For this review, take the finished solid that the model builds, in its own axes (mm). Round coordinates to 2 decimals unless told otherwise and drop trailing zeros. Order: outer loops, then holes, each group sorted by start corner. A loop starts at its lowest first (then second) coordinate and runs counter-clockwise, first axis right, second up. Notation, with made-up numbers: (-13.75, 1) -> (24.25, 1) arc R27 ccw to (24.25, 38) -> close; hole circle Ø11 at (4, -20.75). An arc over 180 degrees is marked (long way). Put each result on its own line as item: value. Start each with the question number.
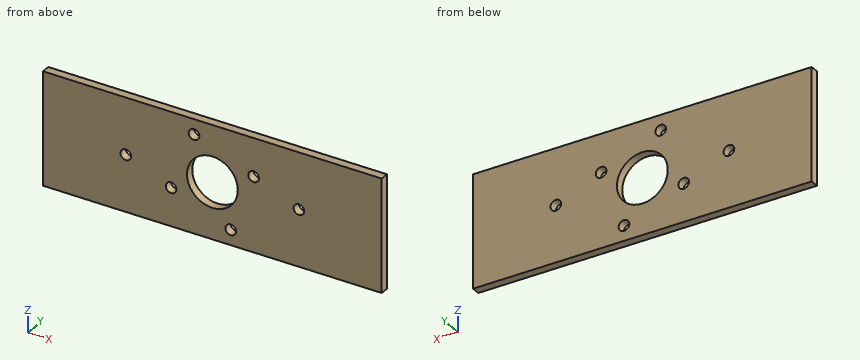
```python
from build123d import *

# Parameters (mm, degrees)
SKETCH1_W                = 190.5
SKETCH1_H                = 63.5
BOSS_EXTRUDE1_DEPTH      = 4.7625
SKETCH3_R                = 14.2875
CUT_EXTRUDE1_DEPTH       = 101.515204851
F_6_0_6_DIAMETER_HOLE1_D = 6


with BuildPart() as part:
    # Sketch1 → Boss-Extrude1 (new body)
    with BuildSketch(Plane(origin=(0, 0, 0), x_dir=(1, 0, 0), z_dir=(0, 1, 0))):
        Rectangle(SKETCH1_W, SKETCH1_H)
    extrude(amount=BOSS_EXTRUDE1_DEPTH)

    # Sketch3 → Cut-Extrude1 (cut, through all)
    with BuildSketch(Plane(origin=(0, 4.7625, 0), x_dir=(1, 0, 0), z_dir=(0, 1, 0))):
        with Locations(Location((0, 0, 0), (0, 0, 270))):
            Circle(SKETCH3_R)
    extrude(amount=-CUT_EXTRUDE1_DEPTH, mode=Mode.SUBTRACT)

    # Ø6.0 (6) Diameter Hole1 (through all)
    with Locations(Plane(origin=(0, 4.7625, 0), x_dir=(1, 0, 0), z_dir=(0, 1, 0))):
        with Locations((-23.209797391, 10.318202609), (-10.318202609, -23.209797391), (10.318202609, 23.209797391), (23.209797391, -10.318202609), (-48.683333333, 0), (48.683333333, 0)):
            Hole(F_6_0_6_DIAMETER_HOLE1_D / 2)


solid = part.part
```
Item 1: Consider section A-A, the plane z = 0. Write out the cut boundary in (x, y).
Item 2: For L1, parallel to Z at x = 1, y = 1.55; L2, parallel to X at y = 3.6, z = 2.5; L3, parallel to X at y = 4.35, z = -10, list the stretches that pass through material, from the lowest coordinate up.
Item 3: Consider section C-C, the plane y = 3.9. Count the separate pieces of the cut face and the enclosed holes in it, plus the area to 3 significant figures.
Item 4: Consider section B-B, the plane x = 0. Write out the cut boundary in (y, z).
Evaluation:
1. outline: (-95.25, 0) -> (-51.68, 0) -> (-51.68, 4.76) -> (-95.25, 4.76) -> close; (-45.68, 0) -> (-14.29, 0) -> (-14.29, 4.76) -> (-45.68, 4.76) -> close; (14.29, 0) -> (45.68, 0) -> (45.68, 4.76) -> (14.29, 4.76) -> close; (51.68, 0) -> (95.25, 0) -> (95.25, 4.76) -> (51.68, 4.76) -> close
2. L1: z = -31.75 to -14.25, 14.25 to 31.75
2. L2: x = -95.25 to -50.34, -47.03 to -14.07, 14.07 to 47.03, 50.34 to 95.25
2. L3: x = -95.25 to -26.19, -20.23 to -10.2, 10.2 to 95.25
3. separate pieces: 1
3. enclosed holes: 7
3. area: 11,300 mm^2
4. outline: (0, -31.75) -> (4.76, -31.75) -> (4.76, -14.29) -> (0, -14.29) -> close; (0, 14.29) -> (4.76, 14.29) -> (4.76, 31.75) -> (0, 31.75) -> close
